from build123d import *

# Parameters (mm, degrees)
SKETCH1_W           = 40
SKETCH1_H           = 20
BOSS_EXTRUDE1_DEPTH = 609.6
SKETCH2_W           = 6
SKETCH2_H           = 609.6
CUT_EXTRUDE1_DEPTH  = 5
SKETCH3_W           = 6
SKETCH3_H           = 609.6
CUT_EXTRUDE2_DEPTH  = 5
SKETCH4_W           = 6
SKETCH4_H           = 609.6
CUT_EXTRUDE3_DEPTH  = 5
SKETCH5_W           = 6
SKETCH5_H           = 609.6
CUT_EXTRUDE4_DEPTH  = 5
SKETCH6_W           = 3
SKETCH6_H           = 609.6
BOSS_EXTRUDE2_DEPTH = 4.75


with BuildPart() as part:
    # Sketch1 → Boss-Extrude1 (new body)
    with BuildSketch(Plane(origin=(0, 0, 0), x_dir=(1, 0, 0), z_dir=(0, 1, 0))):
        with Locations((20, 10)):
            Rectangle(SKETCH1_W, SKETCH1_H)
    extrude(amount=BOSS_EXTRUDE1_DEPTH)

    # Sketch2 → Cut-Extrude1 (cut)
    with BuildSketch(Plane.XY):
        with Locations((10, 304.8)):
            Rectangle(SKETCH2_W, SKETCH2_H)
        with Locations((30, 304.8)):
            Rectangle(SKETCH2_W, SKETCH2_H)
    extrude(amount=-CUT_EXTRUDE1_DEPTH, mode=Mode.SUBTRACT)

    # Sketch3 → Cut-Extrude2 (cut)
    with BuildSketch(Plane.ZY):
        with Locations((-10, 304.8)):
            Rectangle(SKETCH3_W, SKETCH3_H)
    extrude(amount=-CUT_EXTRUDE2_DEPTH, mode=Mode.SUBTRACT)

    # Sketch4 → Cut-Extrude3 (cut)
    with BuildSketch(Plane(origin=(40, 0, 0), x_dir=(0, 0, -1), z_dir=(1, 0, 0))):
        with Locations((10, 304.8)):
            Rectangle(SKETCH4_W, SKETCH4_H)
    extrude(amount=-CUT_EXTRUDE3_DEPTH, mode=Mode.SUBTRACT)

    # Sketch5 → Cut-Extrude4 (cut)
    with BuildSketch(Plane(origin=(0, 0, -20), x_dir=(-1, 0, 0), z_dir=(0, 0, -1))):
        with Locations((-10, 304.8)):
            Rectangle(SKETCH5_W, SKETCH5_H)
    extrude(amount=-CUT_EXTRUDE4_DEPTH, mode=Mode.SUBTRACT)

    # Sketch6 → Boss-Extrude2 (add)
    with BuildSketch(Plane(origin=(0, 0, -20), x_dir=(-1, 0, 0), z_dir=(0, 0, -1))):
        with Locations((-38.5, 304.8)):
            Rectangle(SKETCH6_W, SKETCH6_H)
        with Locations((-1.5, 304.8)):
            Rectangle(SKETCH6_W, SKETCH6_H)
    extrude(amount=BOSS_EXTRUDE2_DEPTH)


solid = part.part
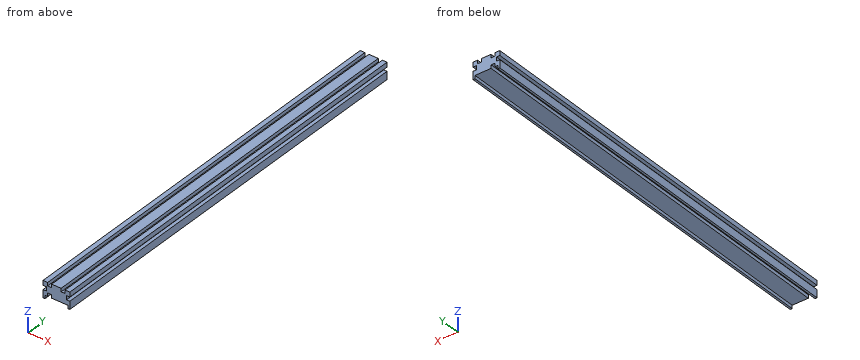
Here's how the part is built. I have some questions about the finished solid (model axes, mm). Round coordinates to 2 decimals unless told otherwise and drop trailing zeros. Write each loop counter-clockwise with the first axis right and the second up, starting at its lowest first coordinate (ties: lowest second). Pieces come first, ordered by that corner, then holes.
1. Suppose I cut it at A-A (y = 226.5). List the corners of the cut face in (x, z) for me.
2. Suppose I cut it at B-B (x = 18). List the corners of the cut face in (y, z) for me.
3. I need wall thicknesses on L1, parallel to X at y = 382, z = -3; L2, parallel to Z at x = 36, y = 110.5; L3, parallel to X at y = 203, z = -20.5. Which ranges of each line are inside material? Lowest first, please.
4. Will these pins go through, and if not, where does the flat tip stop? pin 1 Ø4 at (y, z) = (303, -16.5) entering from -X; pin 2 Ø1.8 at (y, z) = (431, -8.5) entering from -X; pin 3 Ø3 at (x, y) = (10, 284) entering from -Z; pin 4 Ø1.5 at (x, y) = (27.5, 528) entering from -Z.
Answer sheet:
1. outline: (0, -24.75) - (3, -24.75) - (3, -20) - (7, -20) - (7, -15) - (13, -15) - (13, -20) - (37, -20) - (37, -24.75) - (40, -24.75) - (40, -13) - (35, -13) - (35, -7) - (40, -7) - (40, 0) - (33, 0) - (33, -5) - (27, -5) - (27, 0) - (13, 0) - (13, -5) - (7, -5) - (7, 0) - (0, 0) - (0, -7) - (5, -7) - (5, -13) - (0, -13) - close
2. outline: (0, -20) - (609.6, -20) - (609.6, 0) - (0, 0) - close
3. L1: x = 0 to 7, 13 to 27, 33 to 40
3. L2: z = -20 to -13, -7 to 0
3. L3: x = 0 to 3, 37 to 40
4. pin 1: stops at x = 0
4. pin 2: stops at x = 5
4. pin 3: stops at z = -15
4. pin 4: stops at z = -20
